from build123d import *

# Parameters (mm, degrees)
F1_DEPTH = 5.5
F2_R     = 2.5
F3_DEPTH = 15
F4_W     = 10
F4_H     = 5.2
F5_DEPTH = 105


with BuildPart() as f1:
    # F0 (on Top) → F1 (new body, symmetric)
    with BuildSketch(Plane.XY):
        with BuildLine():
            Line((0, 7), (0, 0))
            Line((0, 0), (0, -7))
            Line((0, -7), (48, -7))
            ThreePointArc((48, -7), (52.949747, -4.949747), (55, 0))
            ThreePointArc((55, 0), (52.949747, 4.949747), (48, 7))
            Line((48, 7), (0, 7))
        make_face()
    extrude(amount=F1_DEPTH, both=True)

    # F2 (on face) → F3 (join)
    with BuildSketch(Plane(origin=(0, 0, 0), x_dir=(0, -1, 0), z_dir=(-1, 0, 0))):
        Circle(F2_R)
    extrude(amount=F3_DEPTH)

    # F4 (on face) → F5 (join)
    with BuildSketch(Plane(origin=(-15, 0, 0), x_dir=(0, -1, 0), z_dir=(-1, 0, 0))):
        Rectangle(F4_W, F4_H)
    extrude(amount=F5_DEPTH)


solid = f1.part
Work out the finished part from the listing and answer in its coordinate system (mm). A direction names the side the tool comes from. Give positions to 0.01 mm unless a question says otherwise; leave off trailing zeros. Loops run counter-clockwise (first coordinate to the right, second up) from the corner with the lowest first, then second, coordinate; pieces in that order, holes last. Notation, with made-up numbers: (-22.5, 1.25) - (35.5, 1.25) arc R25 ccw to (35.5, 27.25) - close; hole circle Ø9 at (66.25, -4.5). An arc over 180 degrees is marked (long way). Answer in a Markdown table with one row per item. Add a question column.
Q1. Consider line 1 along Y through (x, z) = (-57, -1); line 2 along X through (y, z) = (4.5, 1); line 3 along Z through (x, y) = (-88.5, -1.25). Determine where each line is inside the solid, lowest interval first.
Q2. Each of these flat-tipped pins is pushed along its axis until it touches: P1, Ø5, axis at x = -47, z = 0.5, coming from the +Y side; P2, Ø6, axis at y = 3.5, z = -2, coming from the +X side; P3, Ø5, axis at x = -75, y = -1, coming from the -Z side. Where does it stop, or does it pass through?
Q3. Determine the mould class of faces 1 (the cylindrical face through (-7.4, 0.54, -2.44)), 2 (the flat face through (0, 0, 3)), 3 (the flat face through (-67, 5, 0)), 4 (the flat face through (-120, 0, 0)) for opening direction X: released by +X, released by -X, zero draft, split by the parting line, or undercut.
Q4. A tool of negligible diameter and unlimited length cuts with its end or side. For faces 5 (the flat face through (-67, 0, 2.6)), 6 (the flat face through (-67, 0, -2.6)), 7 (the flat face through (-67, -5, 0)), from which of +Z, -Z, +X, -X, +Y, -Y can it reach the whole face along a straight path? Write none if from no direction.
Q5. The part is cut by section A-A (z = 0). Determine the outline of the cut face in (x, y), and give its area (3 significant figures).
Solution:
| question | item | result |
|---|---|---|
| 1 | line 1 | y = -5 to 5 |
| 1 | line 2 | x = -120 to -15, 0 to 53.36 |
| 1 | line 3 | z = -2.6 to 2.6 |
| 2 | P1 | stops at y = 5 |
| 2 | P2 | stops at x = 54.98 |
| 2 | P3 | stops at z = -2.6 |
| 3 | face 1 | undercut |
| 3 | face 2 | undercut |
| 3 | face 3 | zero draft |
| 3 | face 4 | released by -X |
| 4 | face 5 | +Z, -X, +Y, -Y |
| 4 | face 6 | -Z, -X, +Y, -Y |
| 4 | face 7 | +Z, -Z, -X, -Y |
| 5 | outline | (-120, -5) - (-15, -5) - (-15, -2.5) - (0, -2.5) - (0, -7) - (48, -7) arc R7 ccw to (55, 0) arc R7 ccw to (48, 7) - (0, 7) - (0, 2.5) - (-15, 2.5) - (-15, 5) - (-120, 5) - close |
| 5 | area | 1,870 mm² |
